from build123d import *

# Parameters (mm, degrees)
F0_R     = 30
F1_DEPTH = 15
F3_DEPTH = 150


with BuildPart() as f1:
    # F0 (on Top) → F1 (new body)
    with BuildSketch(Plane.XY):
        Circle(F0_R)
        with BuildLine():
            ThreePointArc((-16.6170093579, -18.7383297014), (-18.7383297014, -18.7383297014), (-18.7383297014, -16.6170093579))
            Line((-18.7383297014, -16.6170093579), (-8.1317279836, -6.0104076401))
            ThreePointArc((-8.1317279836, -6.0104076401), (-6.0104076401, -6.0104076401), (-6.0104076401, -8.1317279836))
            Line((-6.0104076401, -8.1317279836), (-16.6170093579, -18.7383297014))
        make_face(mode=Mode.SUBTRACT)
        with BuildLine():
            ThreePointArc((1.5, -25), (0, -26.5), (-1.5, -25))
            Line((-1.5, -25), (-1.5, -10))
            ThreePointArc((-1.5, -10), (0, -8.5), (1.5, -10))
            Line((1.5, -10), (1.5, -25))
        make_face(mode=Mode.SUBTRACT)
        with BuildLine():
            ThreePointArc((18.7383297014, -16.6170093579), (18.7383297014, -18.7383297014), (16.6170093579, -18.7383297014))
            Line((16.6170093579, -18.7383297014), (6.0104076401, -8.1317279836))
            ThreePointArc((6.0104076401, -8.1317279836), (6.0104076401, -6.0104076401), (8.1317279836, -6.0104076401))
            Line((8.1317279836, -6.0104076401), (18.7383297014, -16.6170093579))
        make_face(mode=Mode.SUBTRACT)
        with BuildLine():
            ThreePointArc((-25, -1.5), (-26.5, 0), (-25, 1.5))
            Line((-25, 1.5), (-10, 1.5))
            ThreePointArc((-10, 1.5), (-8.5, 0), (-10, -1.5))
            Line((-10, -1.5), (-25, -1.5))
        make_face(mode=Mode.SUBTRACT)
        with BuildLine():
            ThreePointArc((-18.7383297014, 16.6170093579), (-18.7383297014, 18.7383297014), (-16.6170093579, 18.7383297014))
            Line((-16.6170093579, 18.7383297014), (-6.0104076401, 8.1317279836))
            ThreePointArc((-6.0104076401, 8.1317279836), (-6.0104076401, 6.0104076401), (-8.1317279836, 6.0104076401))
            Line((-8.1317279836, 6.0104076401), (-18.7383297014, 16.6170093579))
        make_face(mode=Mode.SUBTRACT)
        with BuildLine():
            ThreePointArc((16.6170093579, 18.7383297014), (18.7383297014, 18.7383297014), (18.7383297014, 16.6170093579))
            Line((18.7383297014, 16.6170093579), (8.1317279836, 6.0104076401))
            ThreePointArc((8.1317279836, 6.0104076401), (6.0104076401, 6.0104076401), (6.0104076401, 8.1317279836))
            Line((6.0104076401, 8.1317279836), (16.6170093579, 18.7383297014))
        make_face(mode=Mode.SUBTRACT)
        with BuildLine():
            ThreePointArc((25, 1.5), (26.5, 0), (25, -1.5))
            Line((25, -1.5), (10, -1.5))
            ThreePointArc((10, -1.5), (8.5, 0), (10, 1.5))
            Line((10, 1.5), (25, 1.5))
        make_face(mode=Mode.SUBTRACT)
        with BuildLine():
            ThreePointArc((-1.5, 25), (0, 26.5), (1.5, 25))
            Line((1.5, 25), (1.5, 10))
            ThreePointArc((1.5, 10), (0, 8.5), (-1.5, 10))
            Line((-1.5, 10), (-1.5, 25))
        make_face(mode=Mode.SUBTRACT)
    extrude(amount=F1_DEPTH)

    # F2 (on face) → F3 (join)
    with BuildSketch(Plane.XY.offset(15)):
        with BuildLine():
            Line((10, 1.5), (12.409673646, 1.5))
            ThreePointArc((12.409673646, 1.5), (11.5484941564, 4.7835429046), (9.8356245592, 7.7143042156))
            Line((9.8356245592, 7.7143042156), (8.1317279836, 6.0104076401))
            ThreePointArc((8.1317279836, 6.0104076401), (6.0104076401, 6.0104076401), (6.0104076401, 8.1317279836))
            Line((6.0104076401, 8.1317279836), (7.7143042156, 9.8356245592))
            ThreePointArc((7.7143042156, 9.8356245592), (4.7835429046, 11.5484941564), (1.5, 12.409673646))
            Line((1.5, 12.409673646), (1.5, 10))
            ThreePointArc((1.5, 10), (0, 8.5), (-1.5, 10))
            Line((-1.5, 10), (-1.5, 12.409673646))
            ThreePointArc((-1.5, 12.409673646), (-4.7835429046, 11.5484941564), (-7.7143042156, 9.8356245592))
            Line((-7.7143042156, 9.8356245592), (-6.0104076401, 8.1317279836))
            ThreePointArc((-6.0104076401, 8.1317279836), (-6.0104076401, 6.0104076401), (-8.1317279836, 6.0104076401))
            Line((-8.1317279836, 6.0104076401), (-9.8356245592, 7.7143042156))
            ThreePointArc((-9.8356245592, 7.7143042156), (-11.5484941564, 4.7835429046), (-12.409673646, 1.5))
            Line((-12.409673646, 1.5), (-10, 1.5))
            ThreePointArc((-10, 1.5), (-8.5, 0), (-10, -1.5))
            Line((-10, -1.5), (-12.409673646, -1.5))
            ThreePointArc((-12.409673646, -1.5), (-11.5484941564, -4.7835429046), (-9.8356245592, -7.7143042156))
            Line((-9.8356245592, -7.7143042156), (-8.1317279836, -6.0104076401))
            ThreePointArc((-8.1317279836, -6.0104076401), (-6.0104076401, -6.0104076401), (-6.0104076401, -8.1317279836))
            Line((-6.0104076401, -8.1317279836), (-7.7143042156, -9.8356245592))
            ThreePointArc((-7.7143042156, -9.8356245592), (-4.7835429046, -11.5484941564), (-1.5, -12.409673646))
            Line((-1.5, -12.409673646), (-1.5, -10))
            ThreePointArc((-1.5, -10), (0, -8.5), (1.5, -10))
            Line((1.5, -10), (1.5, -12.409673646))
            ThreePointArc((1.5, -12.409673646), (4.7835429046, -11.5484941564), (7.7143042156, -9.8356245592))
            Line((7.7143042156, -9.8356245592), (6.0104076401, -8.1317279836))
            ThreePointArc((6.0104076401, -8.1317279836), (6.0104076401, -6.0104076401), (8.1317279836, -6.0104076401))
            Line((8.1317279836, -6.0104076401), (9.8356245592, -7.7143042156))
            ThreePointArc((9.8356245592, -7.7143042156), (11.5484941564, -4.7835429046), (12.409673646, -1.5))
            Line((12.409673646, -1.5), (10, -1.5))
            ThreePointArc((10, -1.5), (8.5, 0), (10, 1.5))
        make_face()
        with BuildLine():
            Line((-10, 1.5), (-12.409673646, 1.5))
            ThreePointArc((-12.409673646, 1.5), (-12.5, 0), (-12.409673646, -1.5))
            Line((-12.409673646, -1.5), (-10, -1.5))
            ThreePointArc((-10, -1.5), (-8.5, 0), (-10, 1.5))
        make_face()
        with BuildLine():
            Line((-6.0104076401, 8.1317279836), (-7.7143042156, 9.8356245592))
            ThreePointArc((-7.7143042156, 9.8356245592), (-8.8388347648, 8.8388347648), (-9.8356245592, 7.7143042156))
            Line((-9.8356245592, 7.7143042156), (-8.1317279836, 6.0104076401))
            ThreePointArc((-8.1317279836, 6.0104076401), (-6.0104076401, 6.0104076401), (-6.0104076401, 8.1317279836))
        make_face()
        with BuildLine():
            Line((1.5, 10), (1.5, 12.409673646))
            ThreePointArc((1.5, 12.409673646), (0, 12.5), (-1.5, 12.409673646))
            Line((-1.5, 12.409673646), (-1.5, 10))
            ThreePointArc((-1.5, 10), (0, 8.5), (1.5, 10))
        make_face()
        with BuildLine():
            Line((8.1317279836, 6.0104076401), (9.8356245592, 7.7143042156))
            ThreePointArc((9.8356245592, 7.7143042156), (8.8388347648, 8.8388347648), (7.7143042156, 9.8356245592))
            Line((7.7143042156, 9.8356245592), (6.0104076401, 8.1317279836))
            ThreePointArc((6.0104076401, 8.1317279836), (6.0104076401, 6.0104076401), (8.1317279836, 6.0104076401))
        make_face()
        with BuildLine():
            ThreePointArc((12.409673646, -1.5), (12.4773979774, -0.7513585779), (12.5, 0))
            ThreePointArc((12.5, 0), (12.4773979774, 0.7513585779), (12.409673646, 1.5))
            Line((12.409673646, 1.5), (10, 1.5))
            ThreePointArc((10, 1.5), (8.5, 0), (10, -1.5))
            Line((10, -1.5), (12.409673646, -1.5))
        make_face()
        with BuildLine():
            ThreePointArc((7.7143042156, -9.8356245592), (8.8388347648, -8.8388347648), (9.8356245592, -7.7143042156))
            Line((9.8356245592, -7.7143042156), (8.1317279836, -6.0104076401))
            ThreePointArc((8.1317279836, -6.0104076401), (6.0104076401, -6.0104076401), (6.0104076401, -8.1317279836))
            Line((6.0104076401, -8.1317279836), (7.7143042156, -9.8356245592))
        make_face()
        with BuildLine():
            ThreePointArc((-1.5, -12.409673646), (0, -12.5), (1.5, -12.409673646))
            Line((1.5, -12.409673646), (1.5, -10))
            ThreePointArc((1.5, -10), (0, -8.5), (-1.5, -10))
            Line((-1.5, -10), (-1.5, -12.409673646))
        make_face()
        with BuildLine():
            ThreePointArc((-9.8356245592, -7.7143042156), (-8.8388347648, -8.8388347648), (-7.7143042156, -9.8356245592))
            Line((-7.7143042156, -9.8356245592), (-6.0104076401, -8.1317279836))
            ThreePointArc((-6.0104076401, -8.1317279836), (-6.0104076401, -6.0104076401), (-8.1317279836, -6.0104076401))
            Line((-8.1317279836, -6.0104076401), (-9.8356245592, -7.7143042156))
        make_face()
    extrude(amount=F3_DEPTH)


solid = f1.part
Can you work these out from the model? Positions are in its coordinate system, mm. A direction names the side the tool comes from. Round coordinates to 2 decimals unless told otherwise and drop trailing zeros. Order: outer loops, then holes, each group sorted by start corner. A loop starts at its lowest first (then second) coordinate and runs counter-clockwise, first axis right, second up. Notation, with made-up numbers: M 3.25,13.5 L 33.25,13.5 A10 ccw 33.25,26.5 Z; hole C -2,-11 d8. An arc over 180 degrees is marked long. Use a Markdown table: item, result.
1) Imagine slicing it at C-C (z = 43.5). List the corners of the cut face in (x, y) for me.
Geometry says:
| item | result |
|---|---|
| outline | C 0,0 d25 |
2) Imagine slicing it at A-A (x = 0). List the corners of the cut face in (y, z) for me.
Geometry says:
| item | result |
|---|---|
| outline | M -30,0 L -26.5,0 L -26.5,15 L -30,15 Z; M -12.5,15 L -8.5,15 L -8.5,0 L 8.5,0 L 8.5,15 L 12.5,15 L 12.5,165 L -12.5,165 Z; M 26.5,0 L 30,0 L 30,15 L 26.5,15 Z |
3) Imagine slicing it at D-D (y = 4). List the corners of the cut face in (x, z) for me, then the cut area to 3 significant figures.
Geometry says:
| item | result |
|---|---|
| outline | M -29.73,0 L 29.73,0 L 29.73,15 L 11.84,15 L 11.84,165 L -11.84,165 L -11.84,15 L -29.73,15 Z |
| area | 4,440 mm² |
4) If we mould it in two halves opening along X, with no side actions, what happens to faces 1 (the face through (-8.5, 0, 7.4)), 2 (the face through (13, -6, 15))? For each: +X half, -X half, draft (parallel to the pull), parting line (faces both ways), or undercut.
Geometry says:
| item | result |
|---|---|
| face 1 | undercut |
| face 2 | draft |
5) I'm going to push flat-ended pins straight in: P1, Ø8, axis at y = -14.5, z = 100.5, coming from the -X side; P2, Ø1.3, axis at x = -7, y = 7, coming from the -Z side; P3, Ø3, axis at x = -15.5, y = 2, coming from the +Z side. Where does each tip first touch, or does it pass through?
Geometry says:
| item | result |
|---|---|
| P1 | stops at x = -6.78 |
| P2 | stops at z = 15 |
| P3 | stops at z = 15 |
6) If I drill on line 1 along X through (y, z) = (6, 8); line 2 along Z through (x, y) = (-23.5, -7); line 3 along Y through (x, z) = (-1.5, 105), over which ranges is the centre line in solid material (lowest first)?
Geometry says:
| item | result |
|---|---|
| line 1 | x = -29.39 to -8.12, -6.02 to 6.02, 8.12 to 29.39 |
| line 2 | z = 0 to 15 |
| line 3 | y = -12.41 to 12.41 |
7) On a 3-axis mill with a long thin cutter (end or side, diameter ignored), from which of +Z, -Z, +X, -X, +Y, -Y can I reach the whole of each face in a straight line? I mean faces 3 (the face through (11.24, 13.36, 7.4)), 4 (the face through (0, 0, 165)). Say none if no direction works.
Geometry says:
| item | result |
|---|---|
| face 3 | -Z |
| face 4 | +Z, +X, -X, +Y, -Y |
8) Imagine slicing it at B-B (y = -14.5). List the corners of the cut face in (x, z) for me, then the cut area to 3 significant figures.
Geometry says:
| item | result |
|---|---|
| outline | M -26.26,0 L -16.62,0 L -16.62,15 L -26.26,15 Z; M -12.38,0 L -1.5,0 L -1.5,15 L -12.38,15 Z; M 1.5,0 L 12.38,0 L 12.38,15 L 1.5,15 Z; M 16.62,0 L 26.26,0 L 26.26,15 L 16.62,15 Z |
| area | 616 mm² |
